The listing builds one solid part. Answer for the finished solid, in the listing's coordinates (mm). Face numbers are marked on the shaded views. Give positions to 0.01 mm unless a question says otherwise; leave off trailing zeros. Write each loop counter-clockwise with the first axis right and the second up, starting at its lowest first coordinate (ties: lowest second). Pieces come first, ordered by that corner, then holes. Notation, with made-up numbers: (-38.5, 9) - (-20.5, 9) arc R24 cw to (-20.5, 32) - close; hole circle Ø11 at (25.25, 73.5). An arc over 180 degrees is marked (long way). Answer in a Markdown table with one row per item. Add a question column.
from build123d import *

# Parameters (mm, degrees)
SKETCH_1_R                   = 44
SKETCH_1_R_2                 = 34
EXTRUDE_1_DEPTH              = 6
SKETCH_2_R                   = 44
SKETCH_2_R_2                 = 31.5
EXTRUDE_2_DEPTH              = 1
HOLE_WIZARD_M4_1_D           = 4.5
HOLE_WIZARD_M4_1_CBORE_D     = 8
HOLE_WIZARD_M4_1_CBORE_DEPTH = 5
PATTERN_CIRCULAR_1_COUNT     = 6
CUT_EXTRUDE_1_DEPTH          = 5
PATTERN_CIRCULAR_2_COUNT     = 6


with BuildPart() as part:
    # 스케치1 → 보스-돌출1 (new body)
    with BuildSketch(Plane(origin=(0, 0, 0), x_dir=(1, 0, 0), z_dir=(0, 1, 0))):
        Circle(SKETCH_1_R)
        Circle(SKETCH_1_R_2, mode=Mode.SUBTRACT)
    extrude(amount=EXTRUDE_1_DEPTH)

    # 스케치2 → 보스-돌출2 (add)
    with BuildSketch(Plane(origin=(0, 6, 0), x_dir=(1, 0, 0), z_dir=(0, 1, 0))):
        Circle(SKETCH_2_R)
        Circle(SKETCH_2_R_2, mode=Mode.SUBTRACT)
    extrude(amount=EXTRUDE_2_DEPTH)

    # M4 육각 소켓 머리 캡 나사용 카운터보어1 (through all)
    with Locations(Plane(origin=(0, 7, 0), x_dir=(1, 0, 0), z_dir=(0, 1, 0))):
        with Locations((0, 39)):
            hole_wizard_m4_1 = CounterBoreHole(HOLE_WIZARD_M4_1_D / 2, HOLE_WIZARD_M4_1_CBORE_D / 2, HOLE_WIZARD_M4_1_CBORE_DEPTH)

    # 원형 패턴1: M4 육각 소켓 머리 캡 나사용 카운터보어1 ×6 about axis
    pattern_circular_1_axis = Axis((0, 0, 0), (0, 1, 0))
    for i in range(1, PATTERN_CIRCULAR_1_COUNT):
        add(hole_wizard_m4_1.rotate(pattern_circular_1_axis, i * 360 / PATTERN_CIRCULAR_1_COUNT), mode=Mode.SUBTRACT)

    # 스케치7 → 컷-돌출1 (cut, symmetric)
    with BuildSketch(Plane(origin=(0, 7, 0), x_dir=(1, 0, 0), z_dir=(0, 1, 0))):
        with BuildLine():
            Line((-4, 39), (-4, 44))
            Line((-4, 44), (4, 44))
            Line((4, 44), (4, 39))
            ThreePointArc((4, 39), (0, 43), (-4, 39))
        make_face()
    cut_extrude_1 = extrude(amount=CUT_EXTRUDE_1_DEPTH, both=True, mode=Mode.SUBTRACT)

    # 원형 패턴2: 컷-돌출1 ×6 about axis
    pattern_circular_2_axis = Axis((0, 0, 0), (0, 1, 0))
    for i in range(1, PATTERN_CIRCULAR_2_COUNT):
        add(cut_extrude_1.rotate(pattern_circular_2_axis, i * 360 / PATTERN_CIRCULAR_2_COUNT), mode=Mode.SUBTRACT)


solid = part.part
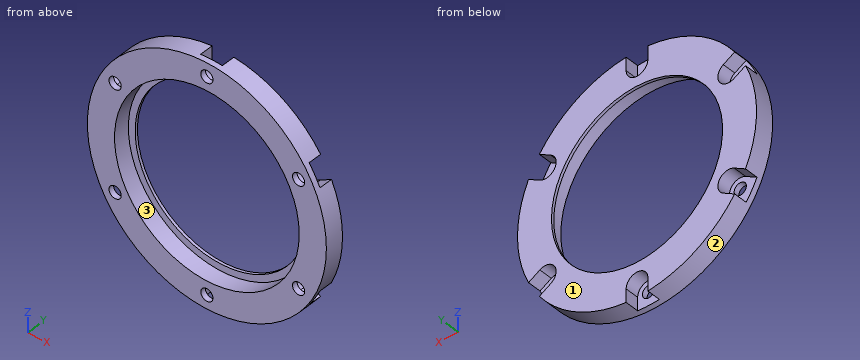
1. Section A-A (z = 0) is taken. Give the vertices of the cut face in (x, y).
2. Section B-B (x = 0) is taken. Give the vertices of the cut face in (y, z).
3. Section C-C (y = 4.75) is taken. Give the vertices of the cut face in (x, z) (3 decimals), and give its area (3 significant figures).
4. Straight lines are drawn through the part: L1, parallel to Z at x = 0, y = 0.95; L2, parallel to X at y = 0.65, z = -19.5 (3 decimals); L3, parallel to X at y = 4, z = 1. For each, find the intervals that lie inside material, in ascending order. Write a range as [from, to].
5. Section D-D (z = 19.5) is taken. Give the vertices of the cut face in (x, y) (3 decimals), and give its area (3 significant figures).
6. The mould has two halves that part along Z. Classify the marked faces 1, 2 and 3: +Z half, -Z half, draft (parallel to the pull), parting line (faces both ways), or undercut.
7. Given pin 1 Ø6 at (x, z) = (-27.5, 14) entering from -Y; pin 2 Ø6 at (x, z) = (-33.77, -19.5) entering from -Y; pin 3 Ø4 at (x, z) = (-1.5, -38.5) entering from +Y; pin 4 Ø3 at (y, z) = (5, 35) entering from -X, each flat-ended and moving along its own axis, determine where each tip first touches the part or whether it passes through.
Geometry check:
| question | item | result |
|---|---|---|
| 1 | outline | (-44, 0) - (-34, 0) - (-34, 6) - (-31.5, 6) - (-31.5, 7) - (-44, 7) - close; (31.5, 6) - (34, 6) - (34, 0) - (44, 0) - (44, 7) - (31.5, 7) - close |
| 2 | outline | (0, -44) - (2, -44) - (2, -41.25) - (0, -41.25) - close; (0, -36.75) - (2, -36.75) - (2, -35) - (7, -35) - (7, -31.5) - (6, -31.5) - (6, -34) - (0, -34) - close; (0, 34) - (6, 34) - (6, 31.5) - (7, 31.5) - (7, 35) - (2, 35) - (2, 36.75) - (0, 36.75) - close; (0, 41.25) - (2, 41.25) - (2, 44) - (0, 44) - close |
| 3 | outline | (-39.947, -18.445) - (-35.775, -16.036) arc R4 cw to (-31.775, -22.964) - (-35.947, -25.373) arc R44 ccw to (-4, -43.818) - (-4, -39) arc R4 cw to (4, -39) - (4, -43.818) arc R44 ccw to (35.947, -25.373) - (31.775, -22.964) arc R4 cw to (35.775, -16.036) - (39.947, -18.445) arc R44 ccw to (39.947, 18.445) - (35.775, 16.036) arc R4 cw to (31.775, 22.964) - (35.947, 25.373) arc R44 ccw to (4, 43.818) - (4, 39) arc R4 cw to (-4, 39) - (-4, 43.818) arc R44 ccw to (-35.947, 25.373) - (-31.775, 22.964) arc R4 cw to (-35.775, 16.036) - (-39.947, 18.445) arc R44 ccw to start; hole circle Ø68 at (0, 0) |
| 3 | area | 2,060 mm² |
| 4 | L1 | [-44, -41.25], [-36.75, -34], [34, 36.75], [41.25, 44] |
| 4 | L2 | [-39.443, -36.025], [-31.525, -27.852], [27.852, 31.525], [36.025, 39.443] |
| 4 | L3 | [-43.99, -33.99], [33.99, 43.99] |
| 5 | outline | (-39.443, 0) - (-36.025, 0) - (-36.025, 2) - (-39.443, 2) - close; (-31.525, 0) - (-27.852, 0) - (-27.852, 6) - (-24.739, 6) - (-24.739, 7) - (-29.775, 7) - (-29.775, 2) - (-31.525, 2) - close; (24.739, 6) - (27.852, 6) - (27.852, 0) - (31.525, 0) - (31.525, 2) - (29.775, 2) - (29.775, 7) - (24.739, 7) - close; (36.025, 0) - (39.443, 0) - (39.443, 2) - (36.025, 2) - close |
| 5 | area | 53.8 mm² |
| 6 | face 1 | draft |
| 6 | face 2 | parting line |
| 6 | face 3 | undercut |
| 7 | pin 1 | y = 6 |
| 7 | pin 2 | y = 0 |
| 7 | pin 3 | y = 2 |
| 7 | pin 4 | x = -28.53 |
